```python
from build123d import *

# Parameters (mm, degrees)
F0_R       = 10.922
F1_DEPTH   = 68.58
F2_R       = 14.9225
F1_FACE1_R = 10.922
F3_DEPTH   = 15.9512
F4_R       = 14.9225
F5_DEPTH   = 14.732
F6_R       = 7.89305
F3_FACE1_R = 14.9225
F7_DEPTH   = 7.9375
F9_DEPTH   = 10.16
F11_DEPTH  = 15.875


with BuildPart() as f1:
    # F0 (on Front) → F1 (new body)
    with BuildSketch(Plane.XZ):
        Circle(F0_R)
    extrude(amount=F1_DEPTH)

    # F2 (on face) + F1_face1 (on face) → F3 (join)
    with BuildSketch(Plane(origin=(0, 0, 0), x_dir=(-1, 0, 0), z_dir=(0, 1, 0))):
        Circle(F2_R)
    with BuildSketch(Plane.XZ.offset(68.58)):
        Circle(F1_FACE1_R)
    extrude(amount=-F3_DEPTH, dir=(0, 1, 0))

    # F4 (on face) → F5 (join)
    with BuildSketch(Plane.XZ.offset(84.5312)):
        Circle(F4_R)
    extrude(amount=-F5_DEPTH)

    # F6 (on face) + F3_face1 (on face) → F7 (join)
    with BuildSketch(Plane.XZ.offset(84.5312)):
        Circle(F6_R)
    with BuildSketch(Plane(origin=(0, 0, 0), x_dir=(-1, 0, 0), z_dir=(0, 1, 0))):
        Circle(F3_FACE1_R)
    extrude(amount=F7_DEPTH, dir=(0, -1, 0))

    # F8 (on face) → F9 (join)
    with BuildSketch(Plane(origin=(0, 0, 0), x_dir=(-1, 0, 0), z_dir=(0, 1, 0))):
        Polygon((-7.7722893238, -13.462), (7.7722893238, -13.462), (15.5445786477, 0), (7.7722893238, 13.462), (-7.7722893238, 13.462), (-15.5445786477, 0), align=None)
    extrude(amount=F9_DEPTH)

    # F10 (on face) → F11 (join)
    with BuildSketch(Plane(origin=(0, 10.16, 0), x_dir=(-1, 0, 0), z_dir=(0, 1, 0))):
        Polygon((-4.0877842434, -7.08025), (4.0877842434, -7.08025), (8.1755684869, 0), (4.0877842434, 7.08025), (-4.0877842434, 7.08025), (-8.1755684869, 0), align=None)
    extrude(amount=F11_DEPTH)


solid = f1.part
```
Design review of the part built by this model. Coordinates are the model's own, in mm. A direction names the side the tool comes from. Give positions to 0.01 mm unless a question says otherwise; leave off trailing zeros. Loops run counter-clockwise (first coordinate to the right, second up) from the corner with the lowest first, then second, coordinate; pieces in that order, holes last. Notation, with made-up numbers: (51, 67) -> (61, 67) arc R30 ccw to (61, 106) -> close; hole circle Ø2 at (-14.5, -26). An arc over 180 degrees is marked (long way). One line per item, written item: value.
Q1. For L1, parallel to Y at x = -8, z = -8; L2, parallel to Y at x = 14.5, z = 3; L3, parallel to X at y = -53, z = -0.5, list the stretches that pass through material, from the lowest coordinate up.
Numbers:
L1: y = -84.53 to -69.8, -15.95 to 10.16
L2: y = -84.53 to -69.8, -15.95 to 0
L3: x = -10.91 to 10.91
Q2. We need section C-C on y = 14.5. Give the boundary of the cut face in (x, z).
Numbers:
outline: (-8.18, 0) -> (-4.09, -7.08) -> (4.09, -7.08) -> (8.18, 0) -> (4.09, 7.08) -> (-4.09, 7.08) -> close
Q3. We need section B-B on x = 0. Give the boundary of the cut face in (y, z) (1 decimal).
Numbers:
outline: (-92.5, -7.9) -> (-84.5, -7.9) -> (-84.5, -14.9) -> (-69.8, -14.9) -> (-69.8, -10.9) -> (-16, -10.9) -> (-16, -14.9) -> (0, -14.9) -> (0, -13.5) -> (10.2, -13.5) -> (10.2, -7.1) -> (26, -7.1) -> (26, 7.1) -> (10.2, 7.1) -> (10.2, 13.5) -> (0, 13.5) -> (0, 14.9) -> (-16, 14.9) -> (-16, 10.9) -> (-69.8, 10.9) -> (-69.8, 14.9) -> (-84.5, 14.9) -> (-84.5, 7.9) -> (-92.5, 7.9) -> close
Q4. We need section A-A on x = 12. Give the boundary of the cut face in (y, z), and give its area (3 significant figures).
Numbers:
outline: (-84.53, -8.87) -> (-69.8, -8.87) -> (-69.8, 8.87) -> (-84.53, 8.87) -> close; (-15.95, -8.87) -> (0, -8.87) -> (0, -6.14) -> (10.16, -6.14) -> (10.16, 6.14) -> (0, 6.14) -> (0, 8.87) -> (-15.95, 8.87) -> close
area: 669 mm^2
Q5. Machinability: for faces 5 (the cylindrical face through (-1.711, -88.444, -7.705)), 6 (the flat face through (12, 0, 7)), 7 (the flat face through (-6.16, 17.99, 3.49)), which of the approach directions +Z, -Z, +X, -X, +Y, -Y give a long, thin tool a straight path to every point of the face, cutting with its end or side? Answer none if there is none.
Numbers:
face 5: -Y
face 6: +Z, +X, +Y
face 7: +Z, -X, +Y
Q6. Draft analysis for pull direction Z (two halves, no side actions). For faces 1 (the flat face through (6, -84.531, -6)), 2 (the flat face through (0, 5, 13.462)), 3 (the cylindrical face through (-14.233, -7.864, 4.482)), 4 (the flat face through (11.71, 5.01, -6.64)), state which applies: pulls with the +Z half, pulls with the -Z half, needs draft (parallel to the pull), parting line crosses it, or undercut.
Numbers:
face 1: needs draft
face 2: pulls with the +Z half
face 3: parting line crosses it
face 4: pulls with the -Z half
Q7. We need section D-D on z = 3. Give the boundary of the cut face in (x, y) (3 decimals), and give its area (3 significant figures).
Numbers:
outline: (-14.618, -84.531) -> (-7.301, -84.531) -> (-7.301, -92.469) -> (7.301, -92.469) -> (7.301, -84.531) -> (14.618, -84.531) -> (14.618, -69.799) -> (10.502, -69.799) -> (10.502, -15.951) -> (14.618, -15.951) -> (14.618, 0) -> (13.813, 0) -> (13.813, 10.16) -> (6.444, 10.16) -> (6.444, 26.035) -> (-6.444, 26.035) -> (-6.444, 10.16) -> (-13.813, 10.16) -> (-13.813, 0) -> (-14.618, 0) -> (-14.618, -15.951) -> (-10.502, -15.951) -> (-10.502, -69.799) -> (-14.618, -69.799) -> close
area: 2,630 mm^2
Q8. For pin 1 Ø1.5 at (x, z) = (2, 9.5) entering from -Y; pin 2 Ø12 at (x, y) = (6.5, -34) entering from +Z; pin 3 Ø5 at (x, z) = (-11.5, -7) entering from +Y, all flat-tipped, find the tip position at first contact; note any pin that passes through.
Numbers:
pin 1: stops at y = -84.53
pin 2: stops at z = 10.91
pin 3: stops at y = 10.16
